```python
from build123d import *

# Parameters (mm, degrees)
F3_D = 8


with BuildPart() as f1:
    # F0 (on Right) → F1 (revolve)
    with BuildSketch(Plane.YZ):
        Polygon((0, 12.5), (0, 0), (20, 0), (20, 12.5), (17.5, 12.5), (17.5, 7.5), (2.5, 7.5), (2.5, 12.5), align=None)
    revolve(axis=Axis((0, 10, 0), (0, 1, 0)))

    # F3 (through all)
    with Locations(Plane.XZ):
        with Locations((0, 0)):
            Hole(F3_D / 2)


solid = f1.part
```
Could you check a few things on this model? Use its own coordinates, in mm. A direction names the side the tool comes from. Coordinates: 2 decimals unless noted, no trailing zeros. Loops run counter-clockwise (first coordinate to the right, second up) from the corner with the lowest first, then second, coordinate; pieces in that order, holes last. Notation, with made-up numbers: M 16.25,12.5 L 43.25,12.5 A36 ccw 43.25,46.5 Z; hole C -15.75,10.5 d11. An arc over 180 degrees is marked long. Put each result on its own line as item: value. Start each with the question number.
(1) Suppose I cut it at D-D on x = 9. Please give me the cut outline in (y, z).
(2) Suppose I cut it at C-C on y = 16.25. Please give me the cut outline in (x, z), then the cut area to 3 significant figures.
(3) I need wall thicknesses on line 1 (Y direction, x = 8.5, z = 3.5); line 2 (Z direction, x = 2.5, y = 13); line 3 (X direction, y = 9.25, z = -1.5). Which ranges of each line are inside material? Lowest first, please. Write a range as from..to.
(4) Suppose I cut it at A-A on z = 0. Please give me the cut outline in (x, y), then the cut area to 3 significant figures.
(5) For faces 1 (the face through (0.33, 9.895, -7.493)), 2 (the face through (3, 0, -3)), which set-ups out of +Z, -Z, +X, -X, +Y, -Y let a thin tool reach every point of the face, with its end or its side?
(6) Suppose I cut it at B-B on x = 0. Please give me the cut outline in (y, z).
(7) Will these pins go through, and if not, where does the flat tip stop? P1, Ø4, axis at x = -8, z = 4, coming from the -Y side; P2, Ø6, axis at y = 9, z = -6.5, coming from the -X side; P3, Ø1.5, axis at y = 16, z = 3, coming from the +X side; P4, Ø7, axis at x = 0, z = 0, coming from the +Y side.
(8) Thinking about a two-plate mould opening in Y: for faces 3 (the face through (3.755, 18.732, 11.923)), 4 (the face through (-8, 17.5, 0)), 5 (the face through (3, 20, 3)), which applies, pulls with the +Y half, pulls with the -Y half, needs draft (parallel to the pull), parting line crosses it, or undercut?
Solutions:
1. outline: M 0,-8.67 L 2.5,-8.67 L 2.5,8.67 L 0,8.67 Z; M 17.5,-8.67 L 20,-8.67 L 20,8.67 L 17.5,8.67 Z
2. outline: C 0,0 d15; hole C 0,0 d8
2. area: 126 mm2
3. line 1: y = 0..2.5, 17.5..20
3. line 2: z = -7.07..-3.12, 3.12..7.07
3. line 3: x = -7.35..-3.71, 3.71..7.35
4. outline: M -12.5,0 L -4,0 L -4,20 L -12.5,20 L -12.5,17.5 L -7.5,17.5 L -7.5,2.5 L -12.5,2.5 Z; M 4,0 L 12.5,0 L 12.5,2.5 L 7.5,2.5 L 7.5,17.5 L 12.5,17.5 L 12.5,20 L 4,20 Z
4. area: 190 mm2
5. face 1: none
5. face 2: +Z, -Z, +X, -X, -Y
6. outline: M 0,-12.5 L 2.5,-12.5 L 2.5,-7.5 L 17.5,-7.5 L 17.5,-12.5 L 20,-12.5 L 20,-4 L 0,-4 Z; M 0,4 L 20,4 L 20,12.5 L 17.5,12.5 L 17.5,7.5 L 2.5,7.5 L 2.5,12.5 L 0,12.5 Z
7. P1: stops at y = 0
7. P2: stops at x = -6.63
7. P3: stops at x = 7.15
7. P4: passes through
8. face 3: needs draft
8. face 4: undercut
8. face 5: pulls with the +Y half
